Print and shaded views of the part. All mm, measured from the part's lowest x, y and z. Round coordinates to 2 decimals unless told otherwise and drop trailing zeros. Write each loop counter-clockwise with the first axis right and the second up, starting at its lowest first coordinate (ties: lowest second). Pieces come first, ordered by that corner, then holes.
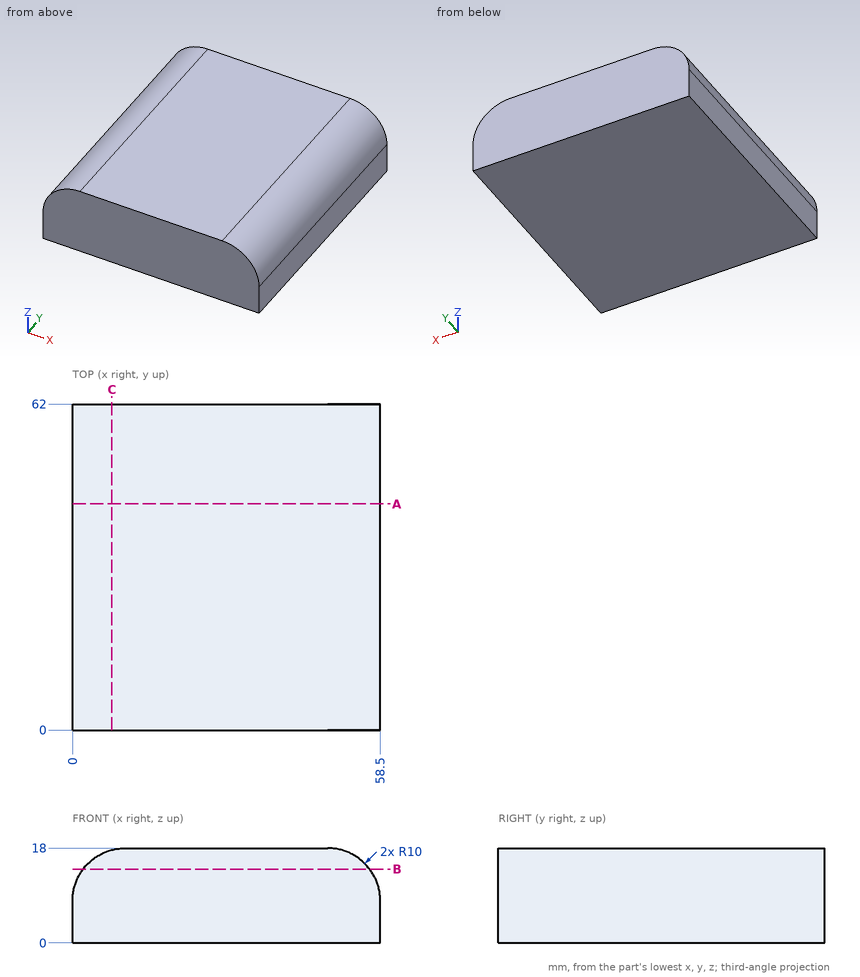
1) Slice it at B-B (z = 14). Write the cut outline in (x, y), plus the area to 3 significant figures.
Results:
outline: (2, 0) - (56.5, 0) - (56.5, 62) - (2, 62) - close
area: 3,380 mm2
2) Slice it at A-A (y = 43). Write the cut outline in (x, z).
Results:
outline: (0, 0) - (58.5, 0) - (58.5, 8) arc R10 ccw to (48.5, 18) - (10, 18) arc R10 ccw to (0, 8) - close
3) Slice it at C-C (x = 7.5). Write the cut outline in (y, z).
Results:
outline: (0, 0) - (62, 0) - (62, 17.68) - (0, 17.68) - close
4) Pin check, flat tips, straight feed: pin 1 Ø2 at (y, z) = (15, 12.5) entering from -X; pin 2 Ø5 at (x, y) = (52, 6.5) entering from +Z; pin 3 Ø5 at (y, z) = (20, 12) entering from -X. Stop position of each tip, or through.
Results:
pin 1: stops at x = 0.63
pin 2: stops at z = 17.95
pin 3: stops at x = 0.11
5) Wall check: L1, parallel to X at y = 27, z = 11.25; L2, parallel to X at y = 49, z = 10.5; L3, parallel to Z at x = 53, y = 6.5. Give the ranges that are in metal, low to high.
Results:
L1: x = 0.54 to 57.96
L2: x = 0.32 to 58.18
L3: z = 0 to 16.93
